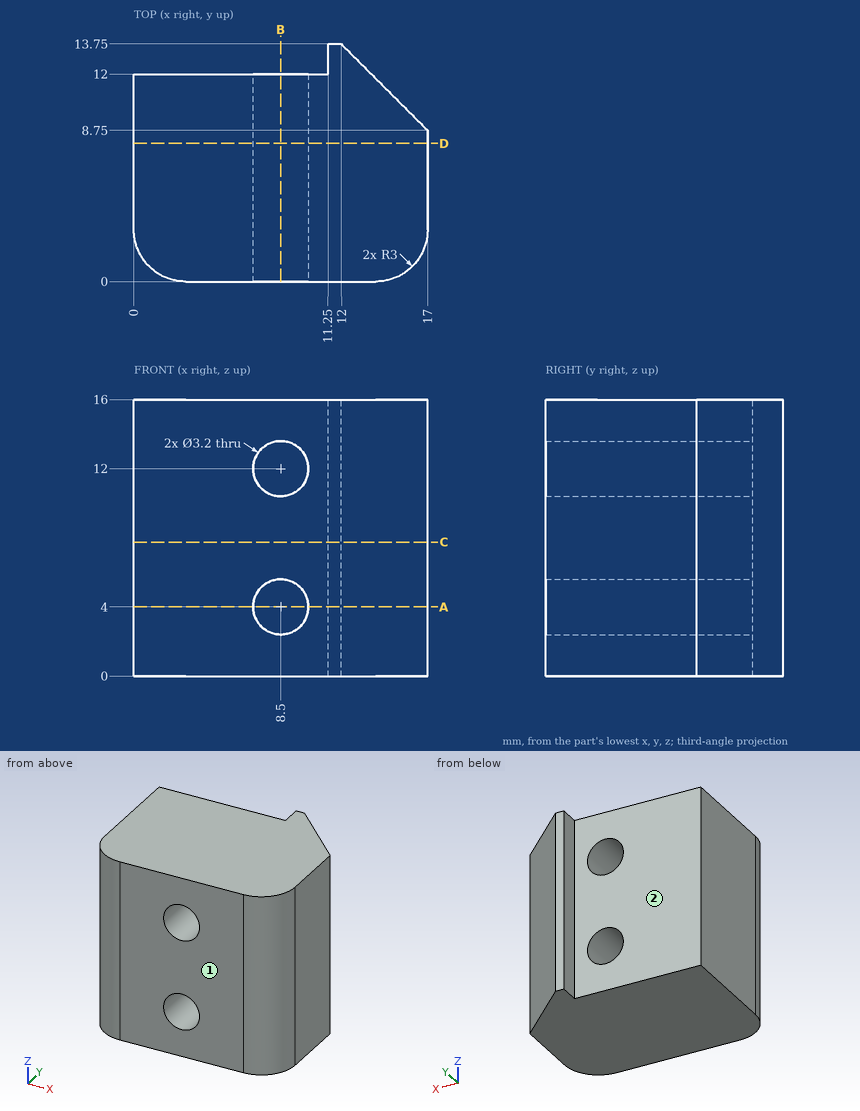
Design review of the part shown in the three views and the two pictorial views. Dimensions are in mm from the part's minimum x, y and z. A direction names the side the tool comes from. Coordinates: 2 decimals unless noted, no trailing zeros. Write each loop counter-clockwise with the first axis right and the second up, starting at its lowest first coordinate (ties: lowest second). Pieces come first, ordered by that corner, then holes.
(1) Wall thickness on probe 1 along Z at (x, y) = (8.5, 6); probe 2 along X at (y, z) = (6.75, 12); probe 3 along Y at (x, z) = (4.75, 0.75): over which ranges is each line inside the solid? List them lowest first.
(2) Add section B-B on x = 8.5. Give the boundary of the cut face in (y, z).
(3) For pin 1 Ø0.5 at (y, z) = (13, 11) entering from -X; pin 2 Ø5 at (x, z) = (8.5, 12) entering from +Y; pin 3 Ø1.9 at (x, z) = (8.5, 4) entering from -Y, all flat-tipped, find the tip position at first contact; note any pin that passes through.
(4) Add section D-D on y = 8. Give the boundary of the cut face in (x, z).
(5) Add section A-A on z = 4. Give the boundary of the cut face in (x, y), then the cut area to 3 significant figures.
(6) Tool access review of the marked faces 1 and 2: name each direction out of +Z, -Z, +X, -X, +Y, -Y from which nothing blocks a thin tool from reaching the whole face with its end or side.
(7) Add section C-C on z = 7.75. Give the boundary of the cut face in (x, y).
Answer sheet:
1. probe 1: z = 0 to 2.4, 5.6 to 10.4, 13.6 to 16
1. probe 2: x = 0 to 6.9, 10.1 to 17
1. probe 3: y = 0 to 12
2. outline: (0, 0) - (12, 0) - (12, 2.4) - (0, 2.4) - close; (0, 5.6) - (12, 5.6) - (12, 10.4) - (0, 10.4) - close; (0, 13.6) - (12, 13.6) - (12, 16) - (0, 16) - close
3. pin 1: stops at x = 11.25
3. pin 2: stops at y = 12
3. pin 3: passes through
4. outline: (0, 0) - (17, 0) - (17, 16) - (0, 16) - close; hole circle Ø3.2 at (8.5, 4); hole circle Ø3.2 at (8.5, 12)
5. outline: (0, 3) arc R3 ccw to (3, 0) - (6.9, 0) - (6.9, 12) - (0, 12) - close; (10.1, 0) - (14, 0) arc R3 ccw to (17, 3) - (17, 8.75) - (12, 13.75) - (11.25, 13.75) - (11.25, 12) - (10.1, 12) - close
5. area: 159 mm2
6. face 1: +Z, -Z, +X, -X, -Y
6. face 2: +Z, -Z, -X, +Y
7. outline: (0, 3) arc R3 ccw to (3, 0) - (14, 0) arc R3 ccw to (17, 3) - (17, 8.75) - (12, 13.75) - (11.25, 13.75) - (11.25, 12) - (0, 12) - close
